Design review of the part shown in the three views and the two pictorial views. Dimensions are in mm from the part's minimum x, y and z. Coordinates: 2 decimals unless noted, no trailing zeros. Order: outer loops, then holes, each group sorted by start corner. A loop starts at its lowest first (then second) coordinate and runs counter-clockwise, first axis right, second up. Notation, with made-up numbers: M -32.75,-20 L -8.75,-20 A15 ccw -8.75,-4 Z; hole C -3,-32.5 d7. An arc over 180 degrees is marked long. Use CSV: the item, a comma, the result in double quotes.
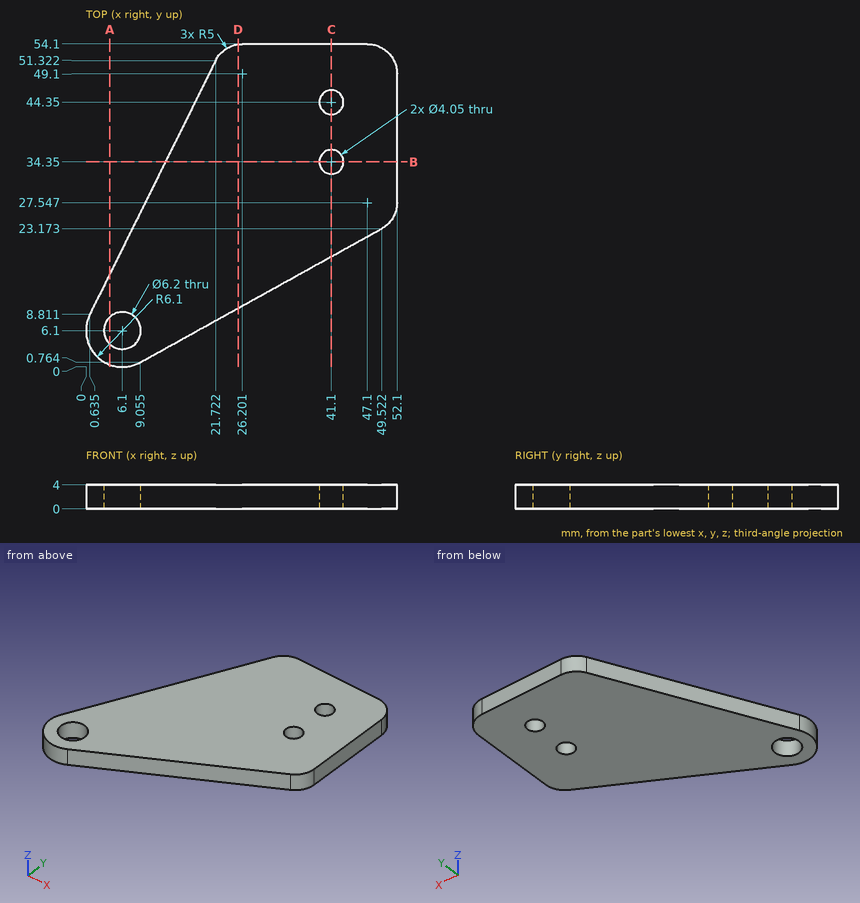
(1) Add section A-A on x = 4. State the section outline as (y, z) points.
The answers:
outline,"M 0.37,0 L 3.82,0 L 3.82,4 L 0.37,4 Z; M 8.38,0 L 15.59,0 L 15.59,4 L 8.38,4 Z"
(2) Clearance check with flat-ended pins moving along their axes: P1, Ø1.5, axis at y = 23.5, z = 3, coming from the -X side; P2, Ø1.5, axis at x = 12.5, z = 1.5, coming from the -Y side (1 decimal). State where each tip first meets the part, or that it passes through.
The answers:
P1,"stops at x = 7.55"
P2,"stops at y = 2.3"
(3) Add section D-D on x = 25.5. State the section outline as (y, z) points, and give its area (3 significant figures).
The answers:
outline,"M 9.87,0 L 54.05,0 L 54.05,4 L 9.87,4 Z"
area,"177 mm2"
(4) Add section B-B on y = 34.35. State the section outline as (x, z) points (1 decimal).
The answers:
outline,"M 13.3,0 L 39.1,0 L 39.1,4 L 13.3,4 Z; M 43.1,0 L 52.1,0 L 52.1,4 L 43.1,4 Z"
(5) Wall thickness on probe 1 along Y at (x, z) = (41.1, 1.45) (1 decimal); probe 2 along Y at (x, z) = (40, 0.4); probe 3 along X at (y, z) = (34.35, 3) (1 decimal): over which ranges is each line inside the solid? List them lowest first.
The answers:
probe 1,"y = 18.5 to 32.3, 36.4 to 42.3, 46.4 to 54.1"
probe 2,"y = 17.9 to 32.65, 36.05 to 42.65, 46.05 to 54.1"
probe 3,"x = 13.3 to 39.1, 43.1 to 52.1"
(6) Add section C-C on x = 41.1. State the section outline as (y, z) points (1 decimal).
The answers:
outline,"M 18.5,0 L 32.3,0 L 32.3,4 L 18.5,4 Z; M 36.4,0 L 42.3,0 L 42.3,4 L 36.4,4 Z; M 46.4,0 L 54.1,0 L 54.1,4 L 46.4,4 Z"
